Answer from the drawing. Dimensions are ordinates in mm from the lowest x, y and z of the part. A direction names the side the tool comes from. Round coordinates to 2 decimals unless told otherwise and drop trailing zeros. Write each loop counter-clockwise with the first axis right and the second up, starting at its lowest first coordinate (ties: lowest second). Pieces come first, ordered by that corner, then holes. Notation, with made-up numbers: (82.25, 3.25) - (98.25, 3.25) arc R23 ccw to (98.25, 18.25) - close; hole circle Ø2 at (16, 6). An arc over 180 degrees is marked (long way). Answer in a Markdown table with one row per item.
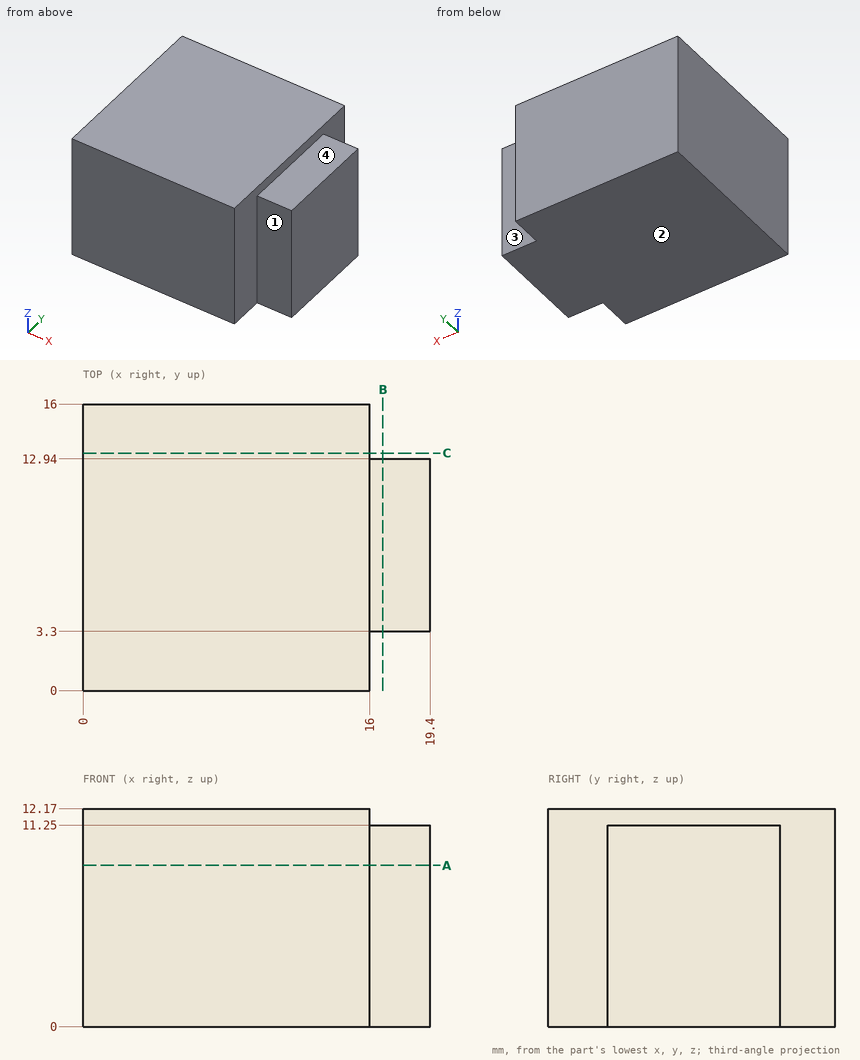
(1) Flat-ended cylindrical pins translate along their axes: pin 1 (2.5 mm diameter, centred on x = 18, z = 7.5, fed in from -Y); pin 2 (3.5 mm diameter, centred on x = 18.5, z = 6.5, fed in from +Y). Find the tip coordinate at first contact, or state that the pin passes through.
Checked values:
| item | result |
|---|---|
| pin 1 | stops at y = 3.3 |
| pin 2 | stops at y = 12.94 |
(2) Section B-B (x = 16.75) is taken. Give the vertices of the cut face in (y, z).
Checked values:
| item | result |
|---|---|
| outline | (3.3, 0) - (12.94, 0) - (12.94, 11.25) - (3.3, 11.25) - close |
(3) Section A-A (z = 9) is taken. Give the vertices of the cut face in (x, y), and give its area (3 significant figures).
Checked values:
| item | result |
|---|---|
| outline | (0, 0) - (16, 0) - (16, 3.3) - (19.4, 3.3) - (19.4, 12.94) - (16, 12.94) - (16, 16) - (0, 16) - close |
| area | 289 mm2 |
(4) Find the intervals of material crossed by line 1 (X direction, y = 3.25, z = 11.75); line 2 (Z direction, x = 18.25, y = 9); line 3 (Y direction, x = 16.25, z = 5), in increasing order.
Checked values:
| item | result |
|---|---|
| line 1 | x = 0 to 16 |
| line 2 | z = 0 to 11.25 |
| line 3 | y = 3.3 to 12.94 |
(5) For the marked faces 1, 2, 3 and 4, determine the directions among +Z, -Z, +X, -X, +Y, -Y from which every point of the face is accessible in a straight line to the end or side of a thin tool.
Checked values:
| item | result |
|---|---|
| face 1 | +Z, -Z, +X, -Y |
| face 2 | -Z, +X, -X, +Y, -Y |
| face 3 | +Z, -Z, +X, +Y |
| face 4 | +Z, +X, +Y, -Y |
(6) Section C-C (y = 13.25) is taken. Give the vertices of the cut face in (x, z), and give its area (3 significant figures).
Checked values:
| item | result |
|---|---|
| outline | (0, 0) - (16, 0) - (16, 12.17) - (0, 12.17) - close |
| area | 195 mm2 |
